The model under review builds one solid part; all positions refer to its coordinate system, in mm. Give positions to 0.01 mm unless a question says otherwise; leave off trailing zeros. Loops run counter-clockwise (first coordinate to the right, second up) from the corner with the lowest first, then second, coordinate; pieces in that order, holes last. Notation, with made-up numbers: M 45.5,-13.75 L 96.5,-13.75 A18 ccw 96.5,-0.75 Z; hole C -7,37.5 d5. An arc over 180 degrees is marked long. One line per item, written item: value. Start each with the question number.
Q1. We need section D-D on x = -11.5. Write out the cut boundary in (y, z).
Q2. We need section B-B on y = 0. Write out the cut boundary in (x, z), plus the area to 3 significant figures.
Q3. For pin 1 (2 mm diameter, centred on x = -10.5, y = 0, fed in from -Z), flat-tipped, find the tip position at first contact; note if it passes through.
Q4. To check wall thickness, follow line 1 along Y through (x, z) = (3, 1.05); line 2 along Z through (x, y) = (3.5, 1.7); line 3 along X through (y, z) = (-0.6, 1.2). State the ranges of each line that lie inside material, in increasing order. Write a range as from..to.
Q5. Mouldability with a two-part tool opening along X and no side actions: class faces 1 (the face through (-13, 0, 1)), 2 (the face through (10, 0, 1)), 3 (the face through (2.261, -0.306, 1.232)) as released by +X, released by -X, zero draft, split by the parting line, or undercut.
Q6. We need section C-C on z = 1.25. Write out the cut boundary in (x, y).
Q7. We need section A-A on x = -3. Write out the cut boundary in (y, z), plus the area to 3 significant figures.
Autodesk Inventor part; units mm, degrees
ref_plane "YZ Plane" through (0, 0, 0) normal (1, 0, 0) x (0, 1, 0)
ref_plane "XZ Plane" through (0, 0, 0) normal (0, 1, 0) x (-1, 0, 0)
ref_plane "XY Plane" through (0, 0, 0) normal (0, 0, 1) x (1, 0, 0)
sketch "スケッチ1" plane through (0, 0, 0) normal (0, 0, 1) x (1, 0, 0)
  line L0 (10, -2) -> (-10, -2)
  line L1 (-10, -2) -> (-10, 2)
  line L2 (-10, 2) -> (10, 2)
  line L3 (10, 2) -> (10, -2)
  line L4 (10, -2) -> (-10, 2) construction
  line L5 (-10, -2) -> (10, 2) construction
  point P0 (0, 0)
  dimension "d0" = 20
  dimension "d1" = 4
extrude "押し出し1" add sketch "スケッチ1" along normal blind 2.5
sketch "スケッチ2" plane through (-10, 2, 0) normal (0, 1, 0) x (1, 0, 0)
  line L0 (0, -1.9) -> (20, -1.9)
  line L1 (20, 0) -> (20, -2.5)
  line L2 (20, -1.9) -> (20, -1.65)
  line L3 (20, -1.65) -> (0, -1.65)
  line L4 (0, -1.65) -> (0, -2.15)
  line L5 (0, -2.15) -> (20, -2.15)
  line L6 (20, -2.15) -> (20, -1.9)
  point P0 (10, 0)
  dimension "d4" = 0.25
  dimension "d5" = 0.5
  dimension "d12" = 20
  dimension "d13" = 20
extrude "押し出し2" cut sketch "スケッチ2" against normal blind 0.5
sketch "スケッチ3" plane through (0, 0, 0) normal (0, 0, -1) x (-1, 0, 0)
  circle A0 centre (3, 0) radius 0.8
  circle A1 centre (-3, 0) radius 0.8
  point P0 (0, 0)
  dimension "d8" = 1.6
  dimension "d9" = 1.6
extrude "押し出し3" cut sketch "スケッチ3" against normal blind 5
sketch "スケッチ5" plane through (-10, -2, 0) normal (-1, 0, 0) x (0, 0, 1)
  line L0 (0, 0) -> (2.5, 0)
  line L1 (0, 4) -> (1.65, 4)
  line L2 (0, 0) -> (0, 4)
  line L3 (1.65, 3.5) -> (1.65, 4)
  line L4 (0, 4) -> (1.65, 4)
  line L5 (1.65, 4) -> (1.65, 3.5)
  line L6 (2.15, 4) -> (2.15, 3.5)
  line L7 (1.65, 3.5) -> (2.15, 3.5)
  line L8 (2.15, 3.5) -> (2.15, 4)
  line L9 (2.5, 0) -> (2.5, 4)
  line L10 (2.15, 4) -> (2.5, 4)
  line L11 (2.5, 4) -> (2.5, 0)
  line L12 (2.5, 0) -> (0, 0)
  point P0 (0, 2)
extrude "押し出し5" add sketch "スケッチ5" along normal blind 3
sketch "スケッチ6" plane through (0, 0, 2.5) normal (0, 0, 1) x (1, 0, 0)
  circle A0 centre (7.5, 0) radius 0.8
  circle A1 centre (-10.5, 0) radius 0.8
  point P0 (0, 0)
  dimension "d20" = 1.6
  dimension "d21" = 1.6
extrude "押し出し6" cut sketch "スケッチ6" against normal blind 3
sketch "スケッチ7" plane through (10, -2, 0) normal (1, 0, 0) x (0, 0, -1)
  line L0 (-2.15, 3.5) -> (-2.15, 4)
  line L1 (-2.15, 4) -> (-2.15, 3.2)
  line L2 (-2.15, 3.2) -> (-1.65, 3.2)
  line L3 (-1.65, 4) -> (-1.65, 3.5)
  line L4 (-1.65, 3.2) -> (-1.65, 4)
  line L5 (-1.65, 4) -> (-2.15, 4)
  point P0 (0, 2)
  dimension "d24" = 0.8
extrude "押し出し7" cut sketch "スケッチ7" against normal blind 30
sketch "スケッチ8" plane through (10, -2, 0) normal (1, 0, 0) x (0, 0, -1)
  line L0 (-1.65, 4) -> (0, 4)
  line L1 (-0.4, 4) -> (-0.4, 3.2)
  line L2 (-2.15, 3.2) -> (-1.65, 3.2)
  line L3 (-0.4, 3.2) -> (-0.9, 3.2)
  line L4 (-0.9, 3.2) -> (-0.9, 4)
  line L5 (-0.9, 4) -> (-0.4, 4)
  point P0 (0, 2)
  dimension "d27" = 0.5
extrude "押し出し8" cut sketch "スケッチ8" against normal blind 30
sketch "スケッチ9" plane through (10, -2, 0) normal (1, 0, 0) x (0, 0, -1)
  line L0 (-2.15, 4) -> (-2.5, 4)
  line L1 (-1.65, 4) -> (-1.65, 3.2)
  line L2 (-2.15, 4) -> (-1.65, 4)
  line L3 (-1.65, 4) -> (-1.65, 3.2)
  line L4 (-1.65, 3.2) -> (-2.15, 3.2)
  line L5 (-2.15, 3.2) -> (-2.15, 4)
  point P0 (0, 2)
extrude "押し出し9" add sketch "スケッチ9" against normal blind 23
properties part number "cutter_stopper" material "ABS プラスチック"
Solved:
1. outline: M -2,0 L 2,0 L 2,0.4 L 1.2,0.4 L 1.2,0.9 L 2,0.9 L 2,2.5 L -2,2.5 Z
2. outline: M -13,0 L -11.3,0 L -11.3,2.5 L -13,2.5 Z; M -9.7,0 L -3.8,0 L -3.8,2.5 L -9.7,2.5 Z; M -2.2,0 L 2.2,0 L 2.2,2.5 L -2.2,2.5 Z; M 3.8,0 L 6.7,0 L 6.7,2.5 L 3.8,2.5 Z; M 8.3,0 L 10,0 L 10,2.5 L 8.3,2.5 Z
2. area: 41.5 mm2
3. pin 1: z = 0
4. line 1: -2..-0.8, 0.8..2
4. line 2: 0..0.4, 0.9..2.5
4. line 3: -13..-11.03, -9.97..-3.53, -2.47..2.47, 3.53..6.97, 8.03..10
5. face 1: released by -X
5. face 2: released by +X
5. face 3: undercut
6. outline: M -13,-2 L 10,-2 L 10,2 L -13,2 Z; hole C -10.5,0 d1.6; hole C -3,0 d1.6; hole C 3,0 d1.6; hole C 7.5,0 d1.6
7. outline: M -2,0 L -0.8,0 L -0.8,2.5 L -2,2.5 Z; M 0.8,0 L 2,0 L 2,0.4 L 1.2,0.4 L 1.2,0.9 L 2,0.9 L 2,2.5 L 0.8,2.5 Z
7. area: 5.60 mm2
